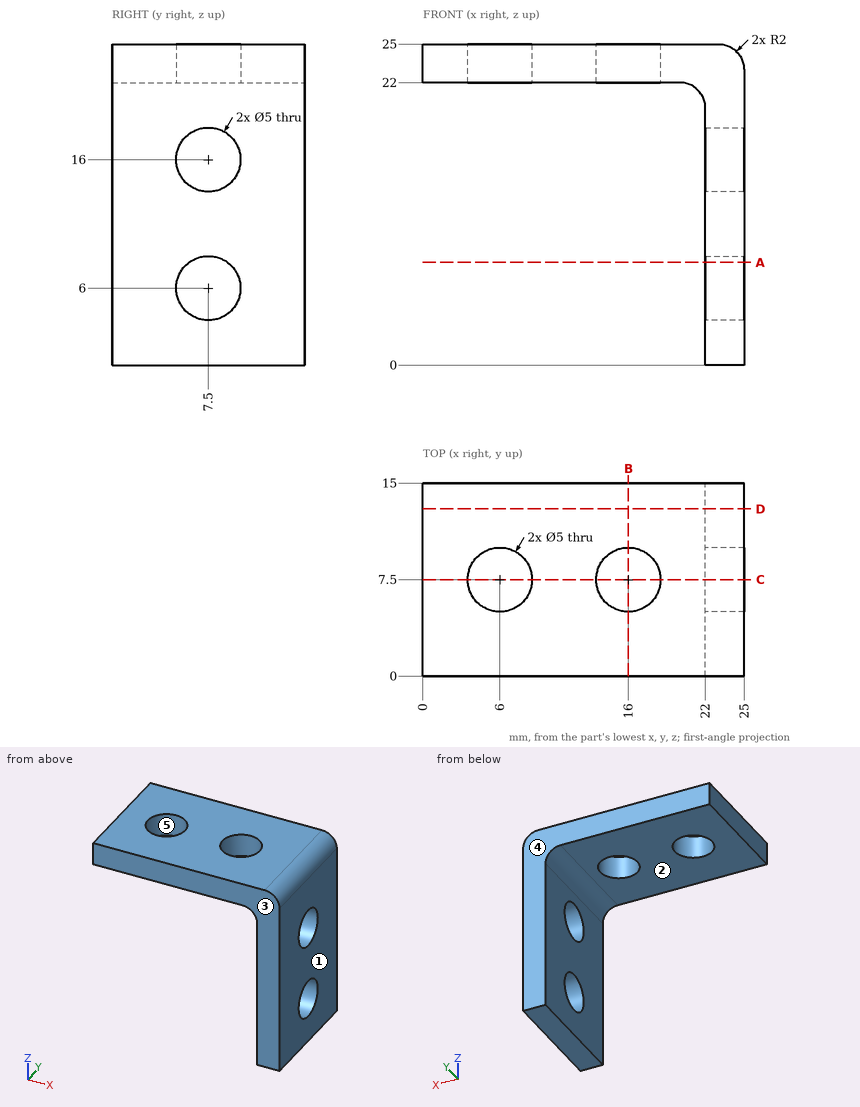
Check sheet for the drawn part. Datum: minimum x, y, z corner. Units: mm. A direction names the side the tool comes from. Round coordinates to 2 decimals unless told otherwise and drop trailing zeros. Order: outer loops, then holes, each group sorted by start corner. A loop starts at its lowest first (then second) coordinate and runs counter-clockwise, first axis right, second up. Notation, with made-up numbers: (-4.5, 27) -> (46.5, 27) arc R23 ccw to (46.5, 38) -> close; hole circle Ø4 at (-25.75, -5). An arc over 180 degrees is marked (long way). Put each result on its own line as item: value. Start each with the question number.
(1) Section check B-B (x = 16). Enter the section's corners in (y, z).
(2) Draft check along Y on the marked faces 3, 4 and 5. Enter one of: +Y half, -Y half, draft (parallel to the pull), parting line (faces both ways), or undercut.
(3) Section check C-C (y = 7.5). Enter the section's corners in (x, z), then the cut area to 3 significant figures.
(4) Section check D-D (y = 13). Enter the section's corners in (x, z), then the cut area to 3 significant figures.
(5) Material ranges on line 1 along Y through (x, z) = (6, 22.7); line 2 along Z through (x, y) = (5.75, 12.75); line 3 along X through (y, z) = (5.5, 23), recorded low to high.
(6) Depth check by flat-ended pin: pin 1 Ø5 at (y, z) = (6.5, 17.5) entering from -X; pin 2 Ø8 at (x, y) = (6, 7.5) entering from +Z; pin 3 Ø6.5 at (x, y) = (16, 7.5) entering from -Z. Enter the tip coordinate at first touch or a pass-through.
(7) Tool access check on the marked faces 1 and 2. Record the directions out of +Z, -Z, +X, -X, +Y, -Y that give a thin tool (end or side, any length) a straight path to the whole face; none if there is none.
(8) Section check A-A (z = 8). Enter the section's corners in (x, y), then the cut area to 3 significant figures.
Completed:
1. outline: (0, 22) -> (5, 22) -> (5, 25) -> (0, 25) -> close; (10, 22) -> (15, 22) -> (15, 25) -> (10, 25) -> close
2. face 3: -Y half
2. face 4: +Y half
2. face 5: undercut
3. outline: (0, 22) -> (3.5, 22) -> (3.5, 25) -> (0, 25) -> close; (8.5, 22) -> (13.5, 22) -> (13.5, 25) -> (8.5, 25) -> close; (18.5, 22) -> (20, 22) arc R2 cw to (22, 20) -> (22, 18.5) -> (25, 18.5) -> (25, 23) arc R2 ccw to (23, 25) -> (18.5, 25) -> close; (22, 0) -> (25, 0) -> (25, 3.5) -> (22, 3.5) -> close; (22, 8.5) -> (25, 8.5) -> (25, 13.5) -> (22, 13.5) -> close
3. area: 81.0 mm2
4. outline: (0, 22) -> (20, 22) arc R2 cw to (22, 20) -> (22, 0) -> (25, 0) -> (25, 23) arc R2 ccw to (23, 25) -> (0, 25) -> close
4. area: 141 mm2
5. line 1: y = 0 to 5, 10 to 15
5. line 2: z = 22 to 25
5. line 3: x = 0 to 4.5, 7.5 to 14.5, 17.5 to 25
6. pin 1: stops at x = 22
6. pin 2: stops at z = 25
6. pin 3: stops at z = 22
7. face 1: +Z, -Z, +X, +Y, -Y
7. face 2: -Z, -X, +Y, -Y
8. outline: (22, 0) -> (25, 0) -> (25, 6) -> (22, 6) -> close; (22, 9) -> (25, 9) -> (25, 15) -> (22, 15) -> close
8. area: 36.0 mm2
